Verification items for this drawing (mm, ordinates from the low corner). A direction names the side the tool comes from. Round coordinates to 2 decimals unless told otherwise and drop trailing zeros. Order: outer loops, then holes, each group sorted by start corner. A loop starts at its lowest first (then second) coordinate and runs counter-clockwise, first axis right, second up. Notation, with made-up numbers: (-4.5, 72.5) - (52.5, 72.5) arc R23 ccw to (52.5, 96.5) - close; hole circle Ø2 at (-29, 57). An arc over 180 degrees is marked (long way). Use a Markdown table: item, result. Add a question column.
(1) Thickness scan on line 1 along X through (y, z) = (27, 29.5); line 2 along Z through (x, y) = (6.87, 36); line 3 along X through (y, z) = (36, 6). Record the ranges inside material, lowest first. Write a range as [from, to].
(2) Gauge pin test, flat end, axial feed: P1, Ø3.5, axis at x = 26.87, z = 6.5, coming from the -Y side. Record the tip position at first contact, or that the pin passes through.
(3) Section check A-A on x = 26.87. Record the boundary of the cut face in (y, z).
(4) Mould release check, pull along X, two halves, no side actions. Record for the marked faces 1, 2, 3 and 4: released by +X, released by -X, zero draft, split by the parting line, or undercut.
(5) Section check C-C on z = 11.5. Record the boundary of the cut face in (x, y).
(6) Section check D-D on y = 24. Record the boundary of the cut face in (x, z), then the cut area to 3 significant figures.
(7) Access from +Z, -Z, +X, -X, +Y, -Y to the whole of each face (thin tool, end or side, straight path). Record for the marked faces 5 and 6.
(8) Section check B-B on z = 26.5. Record the boundary of the cut face in (x, y).
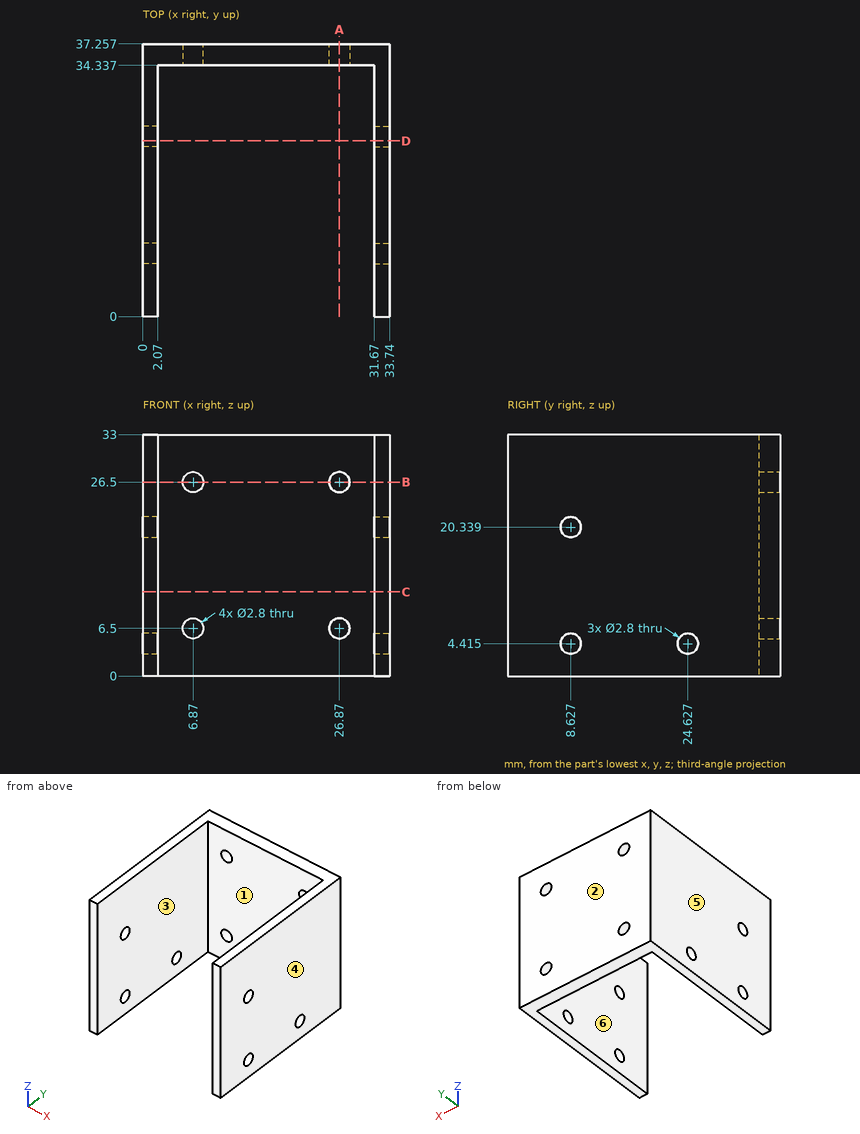
Check sheet entries:
| question | item | result |
|---|---|---|
| 1 | line 1 | x = [0, 2.07], [31.67, 33.74] |
| 1 | line 2 | z = [0, 5.1], [7.9, 25.1], [27.9, 33] |
| 1 | line 3 | x = [0, 5.56], [8.18, 25.56], [28.18, 33.74] |
| 2 | P1 | stops at y = 34.34 |
| 3 | outline | (34.34, 0) - (37.26, 0) - (37.26, 5.1) - (34.34, 5.1) - close; (34.34, 7.9) - (37.26, 7.9) - (37.26, 25.1) - (34.34, 25.1) - close; (34.34, 27.9) - (37.26, 27.9) - (37.26, 33) - (34.34, 33) - close |
| 4 | face 1 | undercut |
| 4 | face 2 | zero draft |
| 4 | face 3 | undercut |
| 4 | face 4 | released by +X |
| 5 | outline | (0, 0) - (2.07, 0) - (2.07, 34.34) - (31.67, 34.34) - (31.67, 0) - (33.74, 0) - (33.74, 37.26) - (0, 37.26) - close |
| 6 | outline | (0, 0) - (2.07, 0) - (2.07, 3.16) - (0, 3.16) - close; (0, 5.67) - (2.07, 5.67) - (2.07, 33) - (0, 33) - close; (31.67, 0) - (33.74, 0) - (33.74, 3.16) - (31.67, 3.16) - close; (31.67, 5.67) - (33.74, 5.67) - (33.74, 33) - (31.67, 33) - close |
| 6 | area | 126 mm2 |
| 7 | face 5 | +Z, -Z, -X, +Y, -Y |
| 7 | face 6 | +Z, -Z, -Y |
| 8 | outline | (0, 0) - (2.07, 0) - (2.07, 34.34) - (5.47, 34.34) - (5.47, 37.26) - (0, 37.26) - close; (8.27, 34.34) - (25.47, 34.34) - (25.47, 37.26) - (8.27, 37.26) - close; (28.27, 34.34) - (31.67, 34.34) - (31.67, 0) - (33.74, 0) - (33.74, 37.26) - (28.27, 37.26) - close |
